Check sheet for the drawn part. Datum: minimum x, y, z corner. Units: mm. Coordinates: 2 decimals unless noted, no trailing zeros. Loops run counter-clockwise (first coordinate to the right, second up) from the corner with the lowest first, then second, coordinate; pieces in that order, holes last.
Q1. Sectioned sample at C-C (z = 1). Enter the section's corners in (x, y).
Q2. Sectioned sample at B-B (x = 35.75). Enter the section's corners in (y, z).
Q3. Go/stop test with a flat-tipped pin: P1, Ø3, axis at x = 3.75, y = 5, coming from the -Z side. Record where the tip stops, or that it passes through.
Q4. Sectioned sample at A-A (y = 5). Enter the section's corners in (x, z).
Q5. Material ranges on probe 1 along X at (y, z) = (5, 0.9); probe 2 along Y at (x, z) = (35.75, 0.4); probe 3 along X at (y, z) = (8.5, 1.75), recorded low to high.
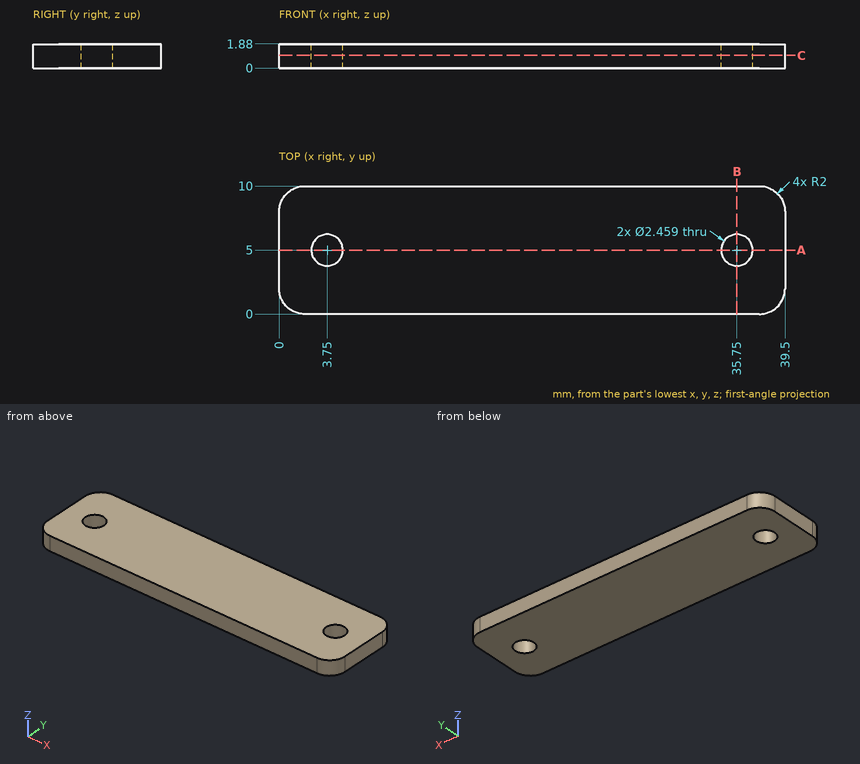
Geometry check:
1. outline: (0, 2) arc R2 ccw to (2, 0) - (37.5, 0) arc R2 ccw to (39.5, 2) - (39.5, 8) arc R2 ccw to (37.5, 10) - (2, 10) arc R2 ccw to (0, 8) - close; hole circle Ø2.46 at (3.75, 5); hole circle Ø2.46 at (35.75, 5)
2. outline: (0, 0) - (3.77, 0) - (3.77, 1.88) - (0, 1.88) - close; (6.23, 0) - (10, 0) - (10, 1.88) - (6.23, 1.88) - close
3. P1: stops at z = 0
4. outline: (0, 0) - (2.52, 0) - (2.52, 1.88) - (0, 1.88) - close; (4.98, 0) - (34.52, 0) - (34.52, 1.88) - (4.98, 1.88) - close; (36.98, 0) - (39.5, 0) - (39.5, 1.88) - (36.98, 1.88) - close
5. probe 1: x = 0 to 2.52, 4.98 to 34.52, 36.98 to 39.5
5. probe 2: y = 0 to 3.77, 6.23 to 10
5. probe 3: x = 0.06 to 39.44
